Source: CAD feature listing. Evaluate the final solid. Frame: model axes, mm. A direction names the side the tool comes from. Give positions to 0.01 mm unless a question says otherwise; leave off trailing zeros. Order: outer loops, then holes, each group sorted by start corner. A loop starts at its lowest first (then second) coordinate and runs counter-clockwise, first axis right, second up.
```python
from build123d import *

# Parameters (mm, degrees)
SKETCH1_W           = 22
SKETCH1_H           = 28
SKETCH1_R           = 1.3
SKETCH1_R_2         = 0.51
BOSS_EXTRUDE1_DEPTH = 1
BOSS_EXTRUDE2_DEPTH = 1.75


with BuildPart() as part:
    # Sketch1 → Boss-Extrude1 (new body)
    with BuildSketch(Plane(origin=(0, 0, 0), x_dir=(1, 0, 0), z_dir=(0, 1, 0))):
        with Locations((11, 14)):
            Rectangle(SKETCH1_W, SKETCH1_H)
        with Locations(Location((2, 2, 0), (0, 0, 270))):
            Circle(SKETCH1_R, mode=Mode.SUBTRACT)
        with Locations(Location((20, 2, 0), (0, 0, 270))):
            Circle(SKETCH1_R, mode=Mode.SUBTRACT)
        with Locations(Location((20, 13, 0), (0, 0, 270))):
            Circle(SKETCH1_R, mode=Mode.SUBTRACT)
        with Locations(Location((2, 13, 0), (0, 0, 270))):
            Circle(SKETCH1_R, mode=Mode.SUBTRACT)
        with Locations(Location((14.81, 24.75, 0), (0, 0, 270))):
            Circle(SKETCH1_R_2, mode=Mode.SUBTRACT)
        with Locations(Location((14.81, 22.21, 0), (0, 0, 270))):
            Circle(SKETCH1_R_2, mode=Mode.SUBTRACT)
        with Locations(Location((12.27, 24.75, 0), (0, 0, 270))):
            Circle(SKETCH1_R_2, mode=Mode.SUBTRACT)
        with Locations(Location((9.73, 24.75, 0), (0, 0, 270))):
            Circle(SKETCH1_R_2, mode=Mode.SUBTRACT)
        with Locations(Location((7.19, 24.75, 0), (0, 0, 270))):
            Circle(SKETCH1_R_2, mode=Mode.SUBTRACT)
        with Locations(Location((12.27, 22.21, 0), (0, 0, 270))):
            Circle(SKETCH1_R_2, mode=Mode.SUBTRACT)
        with Locations(Location((9.73, 22.21, 0), (0, 0, 270))):
            Circle(SKETCH1_R_2, mode=Mode.SUBTRACT)
        with Locations(Location((7.19, 22.21, 0), (0, 0, 270))):
            Circle(SKETCH1_R_2, mode=Mode.SUBTRACT)
    extrude(amount=BOSS_EXTRUDE1_DEPTH)

    # Sketch2 → Boss-Extrude2 (add)
    with BuildSketch(Plane(origin=(0, 1, 0), x_dir=(1, 0, 0), z_dir=(0, 1, 0))):
        with BuildLine():
            Line((9.05, 9.45), (12.95, 9.45))
            ThreePointArc((12.95, 9.45), (13.303553391, 9.303553391), (13.45, 8.95))
            Line((13.45, 8.95), (13.45, 6.05))
            ThreePointArc((13.45, 6.05), (13.303553391, 5.696446609), (12.95, 5.55))
            Line((12.95, 5.55), (9.05, 5.55))
            ThreePointArc((9.05, 5.55), (8.696446609, 5.696446609), (8.55, 6.05))
            Line((8.55, 6.05), (8.55, 8.95))
            ThreePointArc((8.55, 8.95), (8.696446609, 9.303553391), (9.05, 9.45))
        make_face()
    extrude(amount=BOSS_EXTRUDE2_DEPTH)


solid = part.part
```
1) Section query D-D, the plane y = 1.6. Return the cut outline in (x, z), and give its area (3 significant figures).
Report:
outline: (8.55, -8.95) arc R0.5 ccw to (9.05, -9.45) - (12.95, -9.45) arc R0.5 ccw to (13.45, -8.95) - (13.45, -6.05) arc R0.5 ccw to (12.95, -5.55) - (9.05, -5.55) arc R0.5 ccw to (8.55, -6.05) - close
area: 18.9 mm2
2) Section query A-A, the plane z = -13. Return the cut outline in (x, y), and give its area (3 significant figures).
Report:
outline: (0, 0) - (0.7, 0) - (0.7, 1) - (0, 1) - close; (3.3, 0) - (18.7, 0) - (18.7, 1) - (3.3, 1) - close; (21.3, 0) - (22, 0) - (22, 1) - (21.3, 1) - close
area: 16.8 mm2
3) Material intervals for L1, parallel to X at y = 0.3, z = -22.21; L2, parallel to X at y = 0.2, z = -13; L3, parallel to Z at x = 1.75, y = 0.4, sorted ascending.
Report:
L1: x = 0 to 6.68, 7.7 to 9.22, 10.24 to 11.76, 12.78 to 14.3, 15.32 to 22
L2: x = 0 to 0.7, 3.3 to 18.7, 21.3 to 22
L3: z = -28 to -14.28, -11.72 to -3.28, -0.72 to 0
4) Draft query along Z for faces 5 (the flat face through (10.8, 0.5, 0)), 6 (the flat face through (0, 0.5, -13.8)), 7 (the cylindrical face through (7.343, 0.493, -21.724)). Return one class per face: +Z half, -Z half, draft (parallel to the pull), parting line (faces both ways), or undercut.
Report:
face 5: +Z half
face 6: draft
face 7: undercut
5) Section query B-B, the plane x = 2. Return the cut outline in (y, z), and give its area (3 significant figures).
Report:
outline: (0, -28) - (1, -28) - (1, -14.3) - (0, -14.3) - close; (0, -11.7) - (1, -11.7) - (1, -3.3) - (0, -3.3) - close; (0, -0.7) - (1, -0.7) - (1, 0) - (0, 0) - close
area: 22.8 mm2
6) Reachability of faces 1 (the flat face through (11, 2, -9.45)), 2 (the flat face through (11, 2, -5.55)), 3 (the flat face through (22, 0.5, -13.8)), 4 (the flat face through (13.45, 2, -8)) from +Z, -Z, +X, -X, +Y, -Y: full face, straight path, thin tool, end or side. Return the list, or none.
Report:
face 1: -Z, +X, -X, +Y
face 2: +Z, +X, -X, +Y
face 3: +Z, -Z, +X, +Y, -Y
face 4: +Z, -Z, +X, +Y
7) Pin query (flat end, axial travel): pin 1 (0.5 mm diameter, centred on x = 10.5, y = 1.5, fed in from -Z); pin 2 (1.5 mm diameter, centred on y = 1.5, z = -16.5, fed in from -X); pin 3 (6 mm diameter, centred on x = 17, z = -9.5, fed in from +Y); pin 4 (0.9 mm diameter, centred on y = 2, z = -8, fed in from -X). Return the tip coordinate at first contact, or that it passes through.
Report:
pin 1: stops at z = -9.45
pin 2: stops at x = 0
pin 3: stops at y = 1
pin 4: stops at x = 8.55
8) Section query C-C, the plane z = -24.75. Return the cut outline in (x, y).
Report:
outline: (0, 0) - (6.68, 0) - (6.68, 1) - (0, 1) - close; (7.7, 0) - (9.22, 0) - (9.22, 1) - (7.7, 1) - close; (10.24, 0) - (11.76, 0) - (11.76, 1) - (10.24, 1) - close; (12.78, 0) - (14.3, 0) - (14.3, 1) - (12.78, 1) - close; (15.32, 0) - (22, 0) - (22, 1) - (15.32, 1) - close
